Here's the drawing with two shaded views (mm, measured from the low corner). I have some questions. A direction names the side the tool comes from. Round coordinates to 2 decimals unless told otherwise and drop trailing zeros. Loops run counter-clockwise (first coordinate to the right, second up) from the corner with the lowest first, then second, coordinate; pieces in that order, holes last.
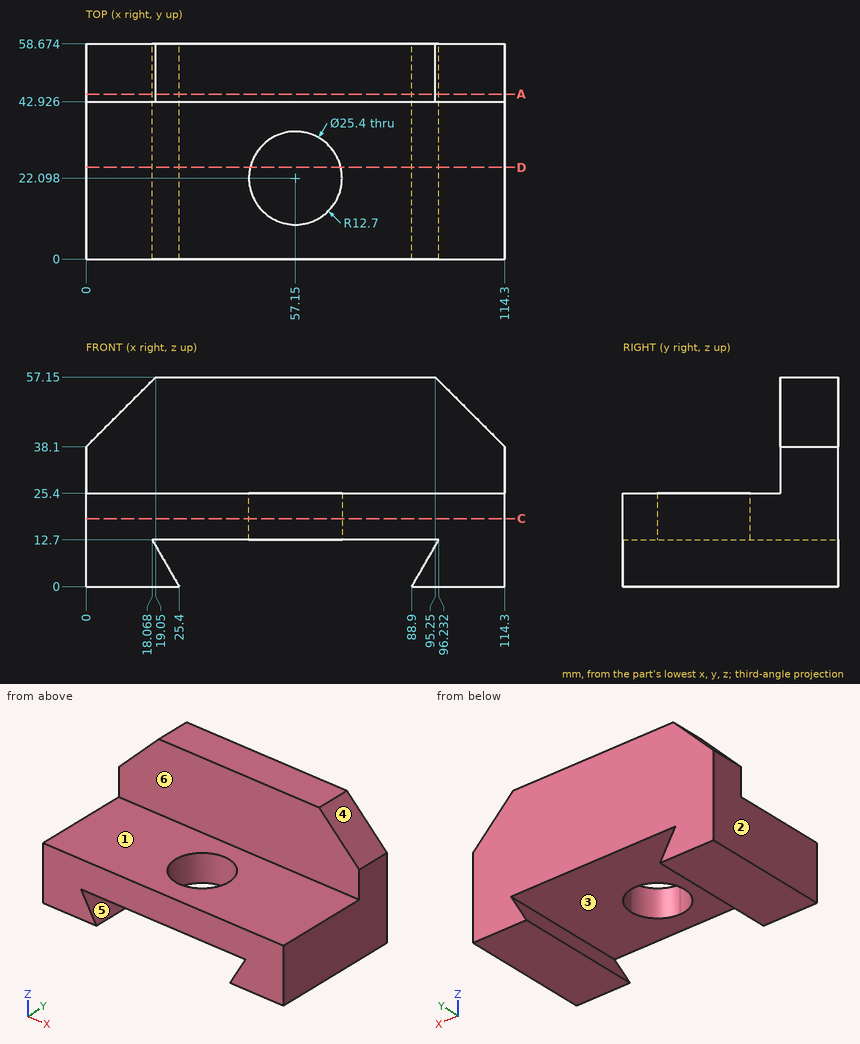
Item 1: We'd pull the mould along X, two halves only. Please class the marked faces 4, 5 and 6: released by +X, released by -X, zero draft, split by the parting line, or undercut.
Results list:
face 4: released by +X
face 5: undercut
face 6: zero draft
Item 2: If we section it at C-C, the plane z = 18.5: Please give me the cut outline in (x, y).
Results list:
outline: (0, 0) - (114.3, 0) - (114.3, 58.67) - (0, 58.67) - close; hole circle Ø25.4 at (57.15, 22.1)
Item 3: If we section it at D-D, the plane y = 25: Please give me the cut outline in (x, z).
Results list:
outline: (0, 0) - (25.4, 0) - (18.07, 12.7) - (44.79, 12.7) - (44.79, 25.4) - (0, 25.4) - close; (69.51, 12.7) - (96.23, 12.7) - (88.9, 0) - (114.3, 0) - (114.3, 25.4) - (69.51, 25.4) - close
Item 4: If we section it at A-A, the plane y = 45: Please give me the cut outline in (x, z), then the cut area to 3 significant figures.
Results list:
outline: (0, 0) - (25.4, 0) - (18.07, 12.7) - (96.23, 12.7) - (88.9, 0) - (114.3, 0) - (114.3, 38.1) - (95.25, 57.15) - (19.05, 57.15) - (0, 38.1) - close
area: 5,270 mm2
Item 5: If I drill on line 1 along Y through (x, z) = (57.15, 22); line 2 along Y through (x, z) = (22, 39.5); line 3 along Z through (x, y) = (27.5, 6.5), over which ranges is the centre line in solid material (lowest first)?
Results list:
line 1: y = 0 to 9.4, 34.8 to 58.67
line 2: y = 42.93 to 58.67
line 3: z = 12.7 to 25.4
Item 6: For the marked faces 1, 2 and 3, which set-ups out of +Z, -Z, +X, -X, +Y, -Y let a thin tool reach every point of the face, with its end or its side?
Results list:
face 1: +Z, +X, -X, -Y
face 2: +Z, -Z, -X, +Y, -Y
face 3: +Y, -Y
Item 7: Will these pins go through, and if not, where does the flat tip stop? pin 1 (12 mm diameter, centred on x = 65.5, z = 43, fed in from -Y); pin 2 (5 mm diameter, centred on x = 96, y = 18.5, fed in from +Z); pin 3 (3 mm diameter, centred on x = 30.5, z = 16.5, fed in from -Y); pin 4 (23 mm diameter, centred on x = 57.15, y = 22.098, fed in from +Z).
Results list:
pin 1: stops at y = 42.93
pin 2: stops at z = 25.4
pin 3: stops at y = 0
pin 4: passes through
